CAD build for the part. Positions are in the model's coordinates, mm. Round coordinates to 2 decimals unless told otherwise and drop trailing zeros. Order: outer loops, then holes, each group sorted by start corner. A loop starts at its lowest first (then second) coordinate and runs counter-clockwise, first axis right, second up.
Autodesk Inventor part; units mm, degrees
ref_plane "YZ Plane" through (0, 0, 0) normal (1, 0, 0) x (0, 1, 0)
ref_plane "XZ Plane" through (0, 0, 0) normal (0, 1, 0) x (-1, 0, 0)
ref_plane "XY Plane" through (0, 0, 0) normal (0, 0, 1) x (1, 0, 0)
sketch "Sketch1" plane through (0, 0, 0) normal (0, 1, 0) x (-1, 0, 0)
  line L0 (54, 54) -> (-54, 54)
  line L1 (-54, 54) -> (-54, -54)
  line L2 (-54, -54) -> (54, -54)
  line L3 (54, -54) -> (54, 54)
  line L4 (54, 54) -> (-54, -54) construction
  line L5 (-54, 54) -> (54, -54) construction
  point P0 (0, 0)
  dimension "d0" = 108
  dimension "d1" = 108
extrude "Extrusion1" add sketch "Sketch1" along normal mid plane 3.175
sketch "Sketch2" plane through (0, 1.5875, 0) normal (0, 1, 0) x (1, 0, 0)
  circle A0 centre (-40, -40) radius 2.5 construction
  circle A1 centre (-46, -46) radius 2
  circle A2 centre (-34, -46) radius 2
  circle A3 centre (-34, -34) radius 2
  circle A4 centre (-46, -34) radius 2
  circle A5 centre (34, -46) radius 2
  circle A6 centre (34, -34) radius 2
  circle A7 centre (46, -34) radius 2
  circle A8 centre (46, -46) radius 2
  circle A9 centre (46, 34) radius 2
  circle A10 centre (34, 34) radius 2
  circle A11 centre (34, 46) radius 2
  circle A12 centre (46, 46) radius 2
  circle A13 centre (-34, 46) radius 2
  circle A14 centre (-34, 34) radius 2
  circle A15 centre (-46, 34) radius 2
  circle A16 centre (-46, 46) radius 2
  point P0 (0, 0)
  dimension "d4" = 5
  dimension "d5" = 40
  dimension "d6" = 40
  dimension "d7" = 4
  dimension "d8" = 6
  dimension "d9" = 6
  dimension "d12" = 360
  dimension "d16" = 360
extrude "Extrusion2" cut sketch "Sketch2" against normal through all
sketch "Sketch3" plane through (0, 1.5875, 0) normal (0, 1, 0) x (1, 0, 0)
  circle A0 centre (0, 0) radius 7
  circle A1 centre (-8, 8) radius 2
  circle A2 centre (-8, -8) radius 2
  circle A3 centre (8, -8) radius 2
  circle A4 centre (8, 8) radius 2
  dimension "d20" = 14
  dimension "d21" = 4
  dimension "d22" = 8
  dimension "d23" = 8
  dimension "d26" = 360
extrude "Extrusion3" cut sketch "Sketch3" against normal through all
properties part number "TurretMotorTopPlate"
1. Cut at C-C, the plane x = 0. Write the cut outline in (y, z).
2. Pin check, flat tips, straight feed: P1, Ø4.5, axis at x = -46, z = 46, coming from the +Y side; P2, Ø2.5, axis at x = -46, z = -46, coming from the +Y side. Stop position of each tip, or through.
3. Mould opens along Z. For faces 1 (the face through (-46, 0, -44)), 2 (the face through (1, 0, -54)), 3 (the face through (13, -1.588, 1)) say: released by +Z, released by -Z, zero draft, split by the parting line, or undercut.
4. Cut at B-B, the plane z = -46. Write the cut outline in (x, y).
5. Drill centre lines: line 1 (X direction, y = 0.15, z = -46); line 2 (X direction, y = 1.4, z = 8). Where is each one in solid material? Low to high.
6. Cut at D-D, the plane x = -34. Write the cut outline in (y, z), and give its area (3 significant figures).
7. Cut at A-A, the plane y = 0.8. Give the number of separate pieces and of enclosed holes in the cut face, and give its area (3 significant figures).
Outcome:
1. outline: (-1.59, -54) - (1.59, -54) - (1.59, -7) - (-1.59, -7) - close; (-1.59, 7) - (1.59, 7) - (1.59, 54) - (-1.59, 54) - close
2. P1: stops at y = 1.59
2. P2: passes through
3. face 1: undercut
3. face 2: released by -Z
3. face 3: zero draft
4. outline: (-54, -1.59) - (-48, -1.59) - (-48, 1.59) - (-54, 1.59) - close; (-44, -1.59) - (-36, -1.59) - (-36, 1.59) - (-44, 1.59) - close; (-32, -1.59) - (32, -1.59) - (32, 1.59) - (-32, 1.59) - close; (36, -1.59) - (44, -1.59) - (44, 1.59) - (36, 1.59) - close; (48, -1.59) - (54, -1.59) - (54, 1.59) - (48, 1.59) - close
5. line 1: x = -54 to -48, -44 to -36, -32 to 32, 36 to 44, 48 to 54
5. line 2: x = -54 to -10, -6 to 6, 10 to 54
6. outline: (-1.59, -54) - (1.59, -54) - (1.59, -48) - (-1.59, -48) - close; (-1.59, -44) - (1.59, -44) - (1.59, -36) - (-1.59, -36) - close; (-1.59, -32) - (1.59, -32) - (1.59, 32) - (-1.59, 32) - close; (-1.59, 36) - (1.59, 36) - (1.59, 44) - (-1.59, 44) - close; (-1.59, 48) - (1.59, 48) - (1.59, 54) - (-1.59, 54) - close
6. area: 292 mm2
7. separate pieces: 1
7. enclosed holes: 21
7. area: 11,300 mm2
